The model under review builds one solid part; all positions refer to its coordinate system, in mm. A direction names the side the tool comes from. Coordinates: 2 decimals unless noted, no trailing zeros. Loops run counter-clockwise (first coordinate to the right, second up) from the corner with the lowest first, then second, coordinate; pieces in that order, holes last. Notation, with made-up numbers: M -39,-2.75 L 2,-2.75 A15 cw 2,14.25 Z; hole C 89.5,84.5 d3. An arc over 180 degrees is marked long. One line per item, written item: value.
```python
from build123d import *

# Parameters (mm, degrees)
SKETCH1_W           = 30
SKETCH1_H           = 20
SKETCH1_R           = 1.65
BOSS_EXTRUDE1_DEPTH = 8
SKETCH3_W           = 4.5
SKETCH3_H           = 20
BOSS_EXTRUDE2_DEPTH = 30
BOSS_EXTRUDE3_DEPTH = 20
SKETCH6_W           = 8.5
SKETCH6_H           = 10
SKETCH6_W_2         = 8.2
CUT_EXTRUDE2_DEPTH  = 30
SKETCH10_R          = 3
CUT_EXTRUDE5_DEPTH  = 4


with BuildPart() as part:
    # Sketch1 → Boss-Extrude1 (new body)
    with BuildSketch(Plane.XY):
        Rectangle(SKETCH1_W, SKETCH1_H)
        with Locations((-10, 0)):
            Circle(SKETCH1_R, mode=Mode.SUBTRACT)
        with Locations((9.999778189, -0.094193404)):
            Circle(SKETCH1_R, mode=Mode.SUBTRACT)
    extrude(amount=BOSS_EXTRUDE1_DEPTH)

    # Sketch3 → Boss-Extrude2 (add)
    with BuildSketch(Plane.XY.offset(8)):
        with Locations((-4.25, 0)):
            Rectangle(SKETCH3_W, SKETCH3_H)
        with Locations((4.55, 0)):
            Rectangle(SKETCH3_W, SKETCH3_H)
    extrude(amount=BOSS_EXTRUDE2_DEPTH)

    # Sketch5 → Boss-Extrude3 (add)
    with BuildSketch(Plane(origin=(0, 10, 0), x_dir=(1, 0, 0), z_dir=(0, 1, 0))):
        Polygon((-15, -8), (-6.5, -38), (-6.5, -8), align=None)
        Polygon((15, -8), (6.8, -8), (6.8, -38), align=None)
    extrude(amount=-BOSS_EXTRUDE3_DEPTH)

    # Sketch6 → Cut-Extrude2 (cut)
    with BuildSketch(Plane.XY.offset(38)):
        with Locations((-10.75, 0)):
            Rectangle(SKETCH6_W, SKETCH6_H)
        with Locations((10.9, 0)):
            Rectangle(SKETCH6_W_2, SKETCH6_H)
    extrude(amount=-CUT_EXTRUDE2_DEPTH, mode=Mode.SUBTRACT)

    # Sketch10 → Cut-Extrude5 (cut)
    with BuildSketch(Plane.XY.offset(8)):
        with Locations((-10, 0)):
            Circle(SKETCH10_R)
        with Locations((9.999778189, -0.094193404)):
            Circle(SKETCH10_R)
    extrude(amount=-CUT_EXTRUDE5_DEPTH, mode=Mode.SUBTRACT)


solid = part.part
```
(1) Add section B-B on y = -4.5. State the section outline as (x, z) points, then the cut area to 3 significant figures.
Checks:
outline: M -15,0 L 15,0 L 15,8 L 6.8,8 L 6.8,38 L 2.3,38 L 2.3,8 L -2,8 L -2,38 L -6.5,38 L -6.5,8 L -15,8 Z
area: 510 mm^2
(2) Tool access review of faces 1 (the face through (-2, 0, 23)), 2 (the face through (-6.5, 0, 23)), 3 (the face through (-8.7, -1.3, 4)), 4 (the face through (6.8, 0, 23)): name each direction out of +Z, -Z, +X, -X, +Y, -Y from which nothing blocks a thin tool from reaching the whole face with its end or side.
Checks:
face 1: +Z, +Y, -Y
face 2: +Z, -X
face 3: +Z
face 4: +Z, +X
(3) Add section C-C on x = -10. State the section outline as (y, z) points.
Checks:
outline: M -10,0 L -1.65,0 L -1.65,4 L -3,4 L -3,8 L -5,8 L -5,25.65 L -10,25.65 Z; M 1.65,0 L 10,0 L 10,25.65 L 5,25.65 L 5,8 L 3,8 L 3,4 L 1.65,4 Z
(4) Add section A-A on z = 26. State the section outline as (x, y) points, then the cut area to 3 significant figures.
Checks:
outline: M -9.9,-10 L -2,-10 L -2,10 L -9.9,10 L -9.9,5 L -6.5,5 L -6.5,-5 L -9.9,-5 Z; M 2.3,-10 L 10.08,-10 L 10.08,-5 L 6.8,-5 L 6.8,5 L 10.08,5 L 10.08,10 L 2.3,10 Z
area: 247 mm^2
(5) Draft analysis for pull direction X (two halves, no side actions). For faces 5 (the face through (0, 0, 8)), 6 (the face through (3, 10, 15)), 7 (the face through (10.843, 7.535, 23.21)), 8 (the face through (-10.81, 7.54, 22.79)), state which applies: pulls with the +X half, pulls with the -X half, needs draft (parallel to the pull), parting line crosses it, or undercut.
Checks:
face 5: undercut
face 6: needs draft
face 7: pulls with the +X half
face 8: pulls with the -X half
(6) Insertion check: pin 1 Ø2 at (x, y) = (10, -0.09) entering from -Z; pin 2 Ø11 at (y, z) = (-2, 19) entering from -X; pin 3 Ø5 at (x, y) = (10.5, -0.5) entering from +Z; pin 4 Ø6 at (y, z) = (-4.5, 16) entering from +X. Each pin has a flat end and moves straight along its axis. Give the tip position at first contact, or say it passes through.
Checks:
pin 1: through
pin 2: x = -13.19
pin 3: z = 8
pin 4: x = 13.62
(7) To check wall thickness, follow L1, parallel to Y at x = -10, z = 5.7; L2, parallel to Y at x = 10, z = 14; L3, parallel to X at y = -2.5, z = 28. State the ranges of each line that lie inside material, in increasing order. Write a range as [from, to].
Checks:
L1: [-10, -3], [3, 10]
L2: [-10, -5], [5, 10]
L3: [-6.5, -2], [2.3, 6.8]
(8) Add section D-D on y = 1. State the section outline as (x, z) points, then the cut area to 3 significant figures.
Checks:
outline: M -15,0 L -11.31,0 L -11.31,4 L -12.83,4 L -12.83,8 L -15,8 Z; M -8.69,0 L 8.76,0 L 8.76,4 L 7.21,4 L 7.21,8 L 6.8,8 L 6.8,38 L 2.3,38 L 2.3,8 L -2,8 L -2,38 L -6.5,38 L -6.5,8 L -7.17,8 L -7.17,4 L -8.69,4 Z; M 11.23,0 L 15,0 L 15,8 L 12.79,8 L 12.79,4 L 11.23,4 Z
area: 445 mm^2
